The model under review builds one solid part; all positions refer to its coordinate system, in mm. Face numbers are marked on the shaded views. A direction names the side the tool comes from. Give positions to 0.01 mm unless a question says otherwise; leave off trailing zeros. Write each loop counter-clockwise with the first axis right and the second up, starting at its lowest first coordinate (ties: lowest second). Pieces come first, ordered by that corner, then holes. Notation, with made-up numbers: (54, 68.5) -> (84, 68.5) arc R13 ccw to (84, 86.5) -> close; hole circle Ø6 at (11, 72). An arc over 180 degrees is marked (long way). Use CSV: the item, a comma, the result in double quotes.
```python
from build123d import *

# Parameters (mm, degrees)
F0_W     = 50.8
F0_H     = 50.8
F1_DEPTH = 50.8
F2_R     = 14.76935
F3_DEPTH = 50.8
F4_R     = 14.855001
F5_DEPTH = 12.7
F6_W     = 26.703719
F6_H     = 20.836989
F7_DEPTH = 12.7


with BuildPart() as f1:
    # F0 (on Front) → F1 (new body)
    with BuildSketch(Plane.XZ):
        with Locations((-30.750444, 29.979647)):
            Rectangle(F0_W, F0_H)
    extrude(amount=F1_DEPTH)

    # F2 (on face) → F3 (cut)
    with BuildSketch(Plane.YZ.offset(-5.350444)):
        with Locations((-26.906017, 28.119825)):
            Circle(F2_R)
    extrude(amount=-F3_DEPTH, mode=Mode.SUBTRACT)

    # F4 (on face) → F5 (join)
    with BuildSketch(Plane(origin=(0, 0, 0), x_dir=(-1, 0, 0), z_dir=(0, 1, 0))):
        with Locations((28.524423, 29.131327)):
            Circle(F4_R)
    extrude(amount=F5_DEPTH)

    # F6 (on face) → F7 (join)
    with BuildSketch(Plane.XZ.offset(50.8)):
        with Locations((-31.963541, 30.446282)):
            Rectangle(F6_W, F6_H)
    extrude(amount=F7_DEPTH)


solid = f1.part
```
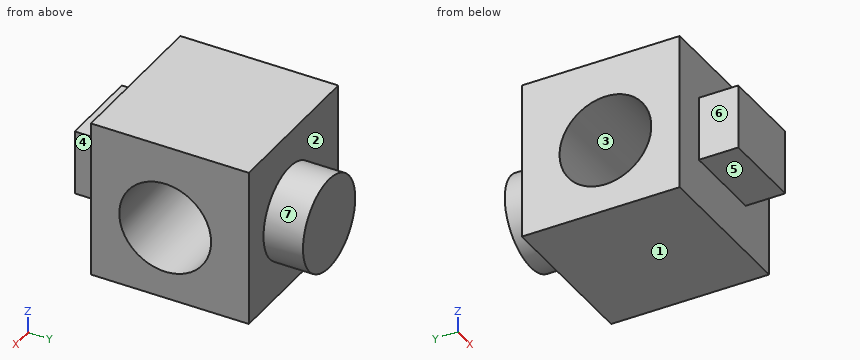
Q1. Consider section A-A (y = -23). Write out the cut boundary in (x, z), then the cut area to 3 significant figures.
Derived:
outline,"(-56.15, 4.58) -> (-5.35, 4.58) -> (-5.35, 13.88) -> (-56.15, 13.88) -> close; (-56.15, 42.36) -> (-5.35, 42.36) -> (-5.35, 55.38) -> (-56.15, 55.38) -> close"
area,"1,130 mm2"
Q2. Consider section B-B (z = 25.5). Write out the cut boundary in (x, y).
Derived:
outline,"(-56.15, -50.8) -> (-45.32, -50.8) -> (-45.32, -63.5) -> (-18.61, -63.5) -> (-18.61, -50.8) -> (-5.35, -50.8) -> (-5.35, -41.44) -> (-56.15, -41.44) -> close; (-56.15, -12.37) -> (-5.35, -12.37) -> (-5.35, 0) -> (-14.12, 0) -> (-14.12, 12.7) -> (-42.93, 12.7) -> (-42.93, 0) -> (-56.15, 0) -> close"
Q3. Consider section C-C (x = -17.5). Write out the cut boundary in (y, z), then the cut area to 3 significant figures.
Derived:
outline,"(-50.8, 4.58) -> (0, 4.58) -> (0, 19.17) -> (12.7, 19.17) -> (12.7, 39.09) -> (0, 39.09) -> (0, 55.38) -> (-50.8, 55.38) -> close; hole circle Ø29.54 at (-26.91, 28.12)"
area,"2,150 mm2"
Q4. The part is to be moulded in two halves that separate along Y. For the marked faces 1, 2 and 3, say which applies: pulls with the +Y half, pulls with the -Y half, needs draft (parallel to the pull), parting line crosses it, or undercut.
Derived:
face 1,"needs draft"
face 2,"pulls with the +Y half"
face 3,"undercut"
Q5. Consider section D-D (x = -23.5). Write out the cut boundary in (y, z).
Derived:
outline,"(-63.5, 20.03) -> (-50.8, 20.03) -> (-50.8, 4.58) -> (0, 4.58) -> (0, 15.15) -> (12.7, 15.15) -> (12.7, 43.11) -> (0, 43.11) -> (0, 55.38) -> (-50.8, 55.38) -> (-50.8, 40.86) -> (-63.5, 40.86) -> close; hole circle Ø29.54 at (-26.91, 28.12)"
Q6. Machinability: for the marked faces 4, 5, 6 and 7, which of the approach directions +Z, -Z, +X, -X, +Y, -Y give a long, thin tool a straight path to every point of the face, cutting with its end or side? Answer none if there is none.
Derived:
face 4,"+Z, -Z, +X, -Y"
face 5,"-Z, +X, -X, -Y"
face 6,"+Z, -Z, -X, -Y"
face 7,"+Y"
Q7. To check wall thickness, follow probe 1 along Z at (x, y) = (-14, -40.5); probe 2 along Y at (x, z) = (-51, 32); probe 3 along Y at (x, z) = (-32, 14.5). State the ranges of each line that lie inside material, in increasing order.
Derived:
probe 1,"z = 4.58 to 22.35, 33.89 to 55.38"
probe 2,"y = -50.8 to -41.16, -12.66 to 0"
probe 3,"y = -50.8 to -32.62, -21.19 to 0"
Q8. Insertion check: pin 1 (10 mm diameter, centred on x = -28, y = -59.5, fed in from +Z); pin 2 (4 mm diameter, centred on y = -55.5, z = 29, fed in from +X); pin 3 (14 mm diameter, centred on x = -27, y = -58.5, fed in from -Z). Each pin has a flat end and moves straight along its axis. Give the tip position at first contact, or say it passes through.
Derived:
pin 1,"stops at z = 40.86"
pin 2,"stops at x = -18.61"
pin 3,"stops at z = 20.03"
